Could you check a few things on this model? Use its own coordinates, in mm. A direction names the side the tool comes from. Give positions to 0.01 mm unless a question says otherwise; leave off trailing zeros. Write each loop counter-clockwise with the first axis right and the second up, starting at its lowest first coordinate (ties: lowest second). Pieces come first, ordered by that corner, then holes. Notation, with made-up numbers: M 65.5,-20 L 121.5,-20 A17 ccw 121.5,-6 Z; hole C 22,26 d2. An arc over 180 degrees is marked long. Write each question's results on one line, items separated by ' | '. Start each with the question number.
from build123d import *

# Parameters (mm, degrees)
BOSS_EXTRUDE1_DEPTH = 2.5


with BuildPart() as part:
    # Sketch1 → Boss-Extrude1 (new body)
    with BuildSketch(Plane.XY):
        with BuildLine():
            ThreePointArc((-8.510567712, 116.344003682), (-2.565917232, 115.465075188), (3.355702363, 114.442428619))
            ThreePointArc((3.355702363, 114.442428619), (4.893623339, 115.566180636), (6.792287095, 115.718152566))
            ThreePointArc((6.792287095, 115.718152566), (-15.794510782, 119.131957807), (-38.598624107, 120.46983672))
            ThreePointArc((-38.598624107, 120.46983672), (-42.143476749, 117.015271661), (-38.68891169, 113.470419019))
            ThreePointArc((-38.68891169, 113.470419019), (-16.523313538, 112.170000716), (5.431053998, 108.851782021))
            ThreePointArc((5.431053998, 108.851782021), (3.750229497, 109.701636852), (2.753244442, 111.299587114))
            ThreePointArc((2.753244442, 111.299587114), (-3.082169507, 112.306976764), (-8.940234626, 113.172980765))
            ThreePointArc((-8.940234626, 113.172980765), (-23.768861657, 114.724233518), (-38.66440506, 115.370260966))
            ThreePointArc((-38.66440506, 115.370260966), (-40.243634801, 116.990765031), (-38.623130736, 118.569994772))
            ThreePointArc((-38.623130736, 118.569994772), (-23.532953855, 117.915525969), (-8.510567712, 116.344003682))
        make_face()
        with BuildLine():
            ThreePointArc((6.42280954, 113.854423418), (7.348162032, 113.300392724), (7.711670546, 112.284967294))
            ThreePointArc((7.711670546, 112.284967294), (7.127095977, 111.048475808), (5.800531553, 110.715511169))
            ThreePointArc((5.800531553, 110.715511169), (4.277812999, 111.012375136), (2.753244442, 111.299587114))
            ThreePointArc((2.753244442, 111.299587114), (3.750229497, 109.701636852), (5.431053998, 108.851782021))
            ThreePointArc((5.431053998, 108.851782021), (8.332913676, 109.580142168), (9.611670546, 112.284967294))
            ThreePointArc((9.611670546, 112.284967294), (8.816495672, 114.506210423), (6.792287095, 115.718152566))
            ThreePointArc((6.792287095, 115.718152566), (4.893623339, 115.566180636), (3.355702363, 114.442428619))
            ThreePointArc((3.355702363, 114.442428619), (4.890181151, 114.153251974), (6.42280954, 113.854423418))
        make_face()
        with BuildLine():
            ThreePointArc((5.800531553, 110.715511169), (4.542214422, 112.596106287), (6.42280954, 113.854423418))
            ThreePointArc((6.42280954, 113.854423418), (4.890181151, 114.153251974), (3.355702363, 114.442428619))
            ThreePointArc((3.355702363, 114.442428619), (2.674256175, 112.943892509), (2.753244442, 111.299587114))
            ThreePointArc((2.753244442, 111.299587114), (4.277812999, 111.012375136), (5.800531553, 110.715511169))
        make_face()
        with BuildLine():
            ThreePointArc((2.753244442, 111.299587114), (2.674256175, 112.943892509), (3.355702363, 114.442428619))
            ThreePointArc((3.355702363, 114.442428619), (-2.565917232, 115.465075188), (-8.510567712, 116.344003682))
            ThreePointArc((-8.510567712, 116.344003682), (-7.13988971, 114.543658766), (-8.940234626, 113.172980765))
            ThreePointArc((-8.940234626, 113.172980765), (-3.082169507, 112.306976764), (2.753244442, 111.299587114))
        make_face()
    extrude(amount=BOSS_EXTRUDE1_DEPTH)


solid = part.part
Q1. If we section it at D-D (y = 110): Please give me the cut outline in (x, z).
Q2. Please list where these lines run through material, in increasing order: line 1 (Y direction, x = 5.5, z = 1); line 2 (Y direction, x = -8, z = 0.95); line 3 (Y direction, x = 1, z = 0.45). Write a range as [from, to].
Q3. I'm going to push flat-ended pins straight in: P1, Ø1, axis at y = 115, z = 1.5, coming from the -X side; P2, Ø3, axis at x = -9, y = 117, coming from the -Z side. Where does each tip first touch, or does it pass through?
Q4. If we section it at B-B (x = -10.5): Please give me the cut outline in (y, z), plus the area to 3 significant figures.
Q5. If we section it at C-C (x = -21): Please give me the cut outline in (y, z).
Q6. If we section it at A-A (z = 0.9): Please give me the cut outline in (x, y), plus the area to 3 significant figures.
Q7. For faces 1 (the face through (-17, 113, 2.5)), 2 (the face through (-23.74, 117.93, 1.23)), which set-ups out of +Z, -Z, +X, -X, +Y, -Y let a thin tool reach every point of the face, with its end or its side?
Q8. If we mould it in two halves opening along X, with no side actions, what happens to faces 3 (the face through (-17, 113, 0)), 4 (the face through (-16.8, 112.2, 1.2)), 5 (the face through (-15.5, 119.1, 1.2)), 6 (the face through (-7.136, 114.579, 1.232))? For each: pulls with the +X half, pulls with the -X half, needs draft (parallel to the pull), parting line crosses it, or undercut.
Determined:
1) outline: M -0.78,0 L 8.76,0 L 8.76,2.5 L -0.78,2.5 Z
2) line 1: y = [108.84, 110.81], [113.76, 115.97] | line 2: y = [111.13, 113.33], [116.18, 118.19] | line 3: y = [109.69, 116.8]
3) P1: stops at x = -41.82 | P2: stops at z = 0
4) outline: M 111.46,0 L 113.38,0 L 113.38,2.5 L 111.46,2.5 Z; M 116.61,0 L 118.52,0 L 118.52,2.5 L 116.61,2.5 Z | area: 9.58 mm²
5) outline: M 112.6,0 L 114.5,0 L 114.5,2.5 L 112.6,2.5 Z; M 117.72,0 L 119.62,0 L 119.62,2.5 L 117.72,2.5 Z
6) outline: M -38.69,113.47 A243 cw 5.43,108.85 A3.5 ccw 6.79,115.72 A250 ccw -38.6,120.47 A3.5 ccw Z; hole M -38.66,115.37 A244.9 cw -8.94,113.17 A1.6 ccw -8.51,116.34 A248.1 ccw -38.62,118.57 A1.6 ccw Z; hole C 6.11,112.28 d3.2 | area: 242 mm²
7) face 1: +Z, +X, -X, +Y, -Y | face 2: +Z, -Z
8) face 3: needs draft | face 4: pulls with the -X half | face 5: pulls with the +X half | face 6: undercut
